from build123d import *


with BuildPart() as f1:
    # F0 (on Front) → F1 (revolve)
    with BuildSketch(Plane.XZ):
        with BuildLine():
            Line((3.3, 3.6), (3.3, 0))
            Line((3.3, 0), (8, 0))
            Line((8, 0), (8, 0.6))
            Line((8, 0.6), (6.26786, 1.206249))
            ThreePointArc((6.26786, 1.206249), (6.073767, 1.352336), (6, 1.583792))
            Line((6, 1.583792), (6, 2.016208))
            ThreePointArc((6, 2.016208), (6.073767, 2.247664), (6.26786, 2.393751))
            Line((6.26786, 2.393751), (8, 3))
            Line((8, 3), (8, 3.6))
            Line((8, 3.6), (3.3, 3.6))
        make_face()
    revolve(axis=Axis((0, 0, 0.328301), (0, 0, -1)))


solid = f1.part
Could you check a few things on this model? Use its own coordinates, in mm. Give positions to 0.01 mm unless a question says otherwise; leave off trailing zeros. Write each loop counter-clockwise with the first axis right and the second up, starting at its lowest first coordinate (ties: lowest second). Pieces come first, ordered by that corner, then holes. Notation, with made-up numbers: (83, 89.5) - (142, 89.5) arc R17 ccw to (142, 101.5) - close; hole circle Ø1 at (8.5, 65). An arc over 180 degrees is marked (long way). Use CSV: the item, a comma, the result in double quotes. Start each with the question number.
Item 1: If we mould it in two halves opening along Z, with no side actions, what happens to faces 1 (the face through (-1.73, 7.81, 0.3)), 2 (the face through (-5.994, -0.264, 1.803)), 3 (the face through (3, 2, 3.6))? For each: pulls with the +Z half, pulls with the -Z half, needs draft (parallel to the pull), parting line crosses it, or undercut.
Item 2: I want a section at D-D, the plane z = 1.8. Please give me the cut outline in (x, y).
Item 3: I'm going to push a flat-ended pin straight in: pin 1 (6 mm diameter, centred on x = 0, y = 0, fed in from +Z). Where does the tip first touch, or does it pass through?
Item 4: If I drill on line 1 along Y through (x, z) = (0, 1.85); line 2 along Z through (x, y) = (5.5, -4), over which ranges is the centre line in solid material (lowest first)?
Item 5: I want a section at C-C, the plane z = 0.3. Please give me the cut outline in (x, y).
Item 6: I want a section at A-A, the plane y = 0. Please give me the cut outline in (x, z), then the cut area to 3 significant figures.
Findings:
1,face 1,"needs draft"
1,face 2,"undercut"
1,face 3,"pulls with the +Z half"
2,outline,"circle Ø12 at (0, 0); hole circle Ø6.6 at (0, 0)"
3,pin 1,"passes through"
4,line 1,"y = -6 to -3.3, 3.3 to 6"
4,line 2,"z = 0 to 1.02, 2.58 to 3.6"
5,outline,"circle Ø16 at (0, 0); hole circle Ø6.6 at (0, 0)"
6,outline,"(-8, 0) - (-3.3, 0) - (-3.3, 3.6) - (-8, 3.6) - (-8, 3) - (-6.27, 2.39) arc R0.4 cw to (-6, 2.02) - (-6, 1.58) arc R0.4 cw to (-6.27, 1.21) - (-8, 0.6) - close; (3.3, 0) - (8, 0) - (8, 0.6) - (6.27, 1.21) arc R0.4 cw to (6, 1.58) - (6, 2.02) arc R0.4 cw to (6.27, 2.39) - (8, 3) - (8, 3.6) - (3.3, 3.6) - close"
6,area,"27.1 mm2"
